Design review of the part built by this model. Coordinates are the model's own, in mm. A direction names the side the tool comes from. Give positions to 0.01 mm unless a question says otherwise; leave off trailing zeros. Write each loop counter-clockwise with the first axis right and the second up, starting at its lowest first coordinate (ties: lowest second). Pieces come first, ordered by that corner, then holes. Notation, with made-up numbers: M 26,16 L 48,16 A9 cw 48,21 Z; hole C 76,74.25 d10. An arc over 180 degrees is marked long. Answer in a Markdown table with one row per item.
```python
from build123d import *

# Parameters (mm, degrees)
BOSS_EXTRUDE4_DEPTH  = 1.5
SKETCH5_W            = 205
SKETCH5_H            = 54
BOSS_EXTRUDE5_DEPTH  = 1.5
SKETCH8_W            = 1.5
SKETCH8_H            = 430
BOSS_EXTRUDE14_DEPTH = 4
SKETCH7_W            = 205
SKETCH7_H            = 54
BOSS_EXTRUDE18_DEPTH = 1.5
SKETCH9_W            = 433
SKETCH9_H            = 54
BOSS_EXTRUDE19_DEPTH = 1.5
SKETCH10_R           = 2.1
CUT_EXTRUDE1_DEPTH   = 10
CUT_EXTRUDE2_START   = -10
SKETCH17_R           = 2.1
CUT_EXTRUDE2_DEPTH   = 10
SKETCH16_R           = 2.1
CUT_EXTRUDE3_DEPTH   = 10
CUT_EXTRUDE4_START   = -10
SKETCH11_R           = 2.1
CUT_EXTRUDE4_DEPTH   = 10
SKETCH12_R           = 2.1
CUT_EXTRUDE5_DEPTH   = 10
SKETCH13_R           = 2.1
CUT_EXTRUDE6_DEPTH   = 10
CUT_EXTRUDE7_START   = -10
SKETCH14_R           = 2.1
CUT_EXTRUDE7_DEPTH   = 10
CUT_EXTRUDE8_START   = -10
SKETCH15_R           = 2.1
CUT_EXTRUDE8_DEPTH   = 10
SKETCH18_W           = 41
SKETCH18_H           = 21.003646253
CUT_EXTRUDE9_DEPTH   = 10
SKETCH21_W           = 53
SKETCH21_H           = 58
CUT_EXTRUDE12_DEPTH  = 10
SKETCH23_W           = 7
SKETCH23_H           = 18
CUT_EXTRUDE14_DEPTH  = 31
SKETCH24_W           = 7
SKETCH24_H           = 18
CUT_EXTRUDE15_DEPTH  = 31


with BuildPart() as part:
    # Sketch4 → Boss-Extrude4 (new body)
    with BuildSketch(Plane(origin=(0, 0, 0), x_dir=(1, 0, 0), z_dir=(0, 1, 0))):
        Polygon((124.01347733, 430), (329.01347733, 430), (329.01347733, 0), (124.01347733, 0), (124.01347733, 200), (124.01347733, 365), align=None)
    extrude(amount=BOSS_EXTRUDE4_DEPTH)

    # Sketch5 → Boss-Extrude5 (add)
    with BuildSketch(Plane.XY):
        with Locations((226.51347733, -25.5)):
            Rectangle(SKETCH5_W, SKETCH5_H)
    extrude(amount=BOSS_EXTRUDE5_DEPTH)

    # Sketch8 → Boss-Extrude14 (add)
    with BuildSketch(Plane(origin=(0, 1.5, 0), x_dir=(1, 0, 0), z_dir=(0, 1, 0))):
        with Locations((328.26347733, 215)):
            Rectangle(SKETCH8_W, SKETCH8_H)
    extrude(amount=BOSS_EXTRUDE14_DEPTH)

    # Sketch7 → Boss-Extrude18 (add)
    with BuildSketch(Plane(origin=(0, 0, -430), x_dir=(-1, 0, 0), z_dir=(0, 0, -1))):
        with Locations((-226.51347733, -25.5)):
            Rectangle(SKETCH7_W, SKETCH7_H)
    extrude(amount=BOSS_EXTRUDE18_DEPTH)

    # Sketch9 → Boss-Extrude19 (add)
    with BuildSketch(Plane.ZY.offset(-124.01347733)):
        with Locations((-215, -25.5)):
            Rectangle(SKETCH9_W, SKETCH9_H)
    extrude(amount=BOSS_EXTRUDE19_DEPTH)

    # Sketch10 → Cut-Extrude1 (cut)
    with BuildSketch(Plane(origin=(0, 0, -431.5), x_dir=(-1, 0, 0), z_dir=(0, 0, -1))):
        with Locations((-154.01347733, -42.5)):
            Circle(SKETCH10_R)
    extrude(amount=-CUT_EXTRUDE1_DEPTH, mode=Mode.SUBTRACT)

    # Sketch17 → Cut-Extrude2 (cut)
    with BuildSketch(Plane.XY.offset(1.5).offset(CUT_EXTRUDE2_START)):
        with Locations(Location((154.01347733, -42.5, 0), (0, 0, 180))):
            Circle(SKETCH17_R)
    extrude(amount=CUT_EXTRUDE2_DEPTH, mode=Mode.SUBTRACT)

    # Sketch16 → Cut-Extrude3 (cut)
    with BuildSketch(Plane.XY.offset(1.5)):
        with Locations((134.023652304, -42.521836229)):
            Circle(SKETCH16_R)
    extrude(amount=-CUT_EXTRUDE3_DEPTH, mode=Mode.SUBTRACT)

    # Sketch11 → Cut-Extrude4 (cut)
    with BuildSketch(Plane(origin=(0, 0, -431.5), x_dir=(-1, 0, 0), z_dir=(0, 0, -1)).offset(CUT_EXTRUDE4_START)):
        with Locations(Location((-134.023652304, -42.521836229, 0), (0, 0, 180))):
            Circle(SKETCH11_R)
    extrude(amount=CUT_EXTRUDE4_DEPTH, mode=Mode.SUBTRACT)

    # Sketch12 → Cut-Extrude5 (cut)
    with BuildSketch(Plane(origin=(0, 0, -431.5), x_dir=(-1, 0, 0), z_dir=(0, 0, -1))):
        with Locations((-134.017306734, -22.477341223)):
            Circle(SKETCH12_R)
    extrude(amount=-CUT_EXTRUDE5_DEPTH, mode=Mode.SUBTRACT)

    # Sketch13 → Cut-Extrude6 (cut)
    with BuildSketch(Plane(origin=(0, 0, -431.5), x_dir=(-1, 0, 0), z_dir=(0, 0, -1))):
        with Locations((-154.003183789, -22.514424589)):
            Circle(SKETCH13_R)
    extrude(amount=-CUT_EXTRUDE6_DEPTH, mode=Mode.SUBTRACT)

    # Sketch14 → Cut-Extrude7 (cut)
    with BuildSketch(Plane.XY.offset(1.5).offset(CUT_EXTRUDE7_START)):
        with Locations(Location((134.017306734, -22.477341223, 0), (0, 0, 180))):
            Circle(SKETCH14_R)
    extrude(amount=CUT_EXTRUDE7_DEPTH, mode=Mode.SUBTRACT)

    # Sketch15 → Cut-Extrude8 (cut)
    with BuildSketch(Plane.XY.offset(1.5).offset(CUT_EXTRUDE8_START)):
        with Locations(Location((154.003183789, -22.514424589, 0), (0, 0, 180))):
            Circle(SKETCH15_R)
    extrude(amount=CUT_EXTRUDE8_DEPTH, mode=Mode.SUBTRACT)

    # Sketch18 → Cut-Extrude9 (cut)
    with BuildSketch(Plane(origin=(0, 1.5, 0), x_dir=(1, 0, 0), z_dir=(0, 1, 0))):
        with Locations((144.235269619, 254.779446877)):
            Rectangle(SKETCH18_W, SKETCH18_H)
    extrude(amount=-CUT_EXTRUDE9_DEPTH, mode=Mode.SUBTRACT)

    # Sketch21 → Cut-Extrude12 (cut)
    with BuildSketch(Plane(origin=(0, 1.5, 0), x_dir=(1, 0, 0), z_dir=(0, 1, 0))):
        with Locations((190.51347733, 360.765424222)):
            Rectangle(SKETCH21_W, SKETCH21_H)
    extrude(amount=-CUT_EXTRUDE12_DEPTH, mode=Mode.SUBTRACT)

    # Sketch23 → Cut-Extrude14 (cut)
    with BuildSketch(Plane.XY.offset(1.5)):
        with Locations((325.51347733, -3.5)):
            Rectangle(SKETCH23_W, SKETCH23_H)
    extrude(amount=-CUT_EXTRUDE14_DEPTH, mode=Mode.SUBTRACT)

    # Sketch24 → Cut-Extrude15 (cut)
    with BuildSketch(Plane(origin=(0, 0, -431.5), x_dir=(-1, 0, 0), z_dir=(0, 0, -1))):
        with Locations((-325.51347733, -3.5)):
            Rectangle(SKETCH24_W, SKETCH24_H)
    extrude(amount=-CUT_EXTRUDE15_DEPTH, mode=Mode.SUBTRACT)


solid = part.part
```
1) Insertion check: P1, Ø5, axis at y = -3, z = -56.5, coming from the +X side; P2, Ø15.5, axis at y = -7, z = -422.5, coming from the +X side; P3, Ø5, axis at x = 241.5, z = -65, coming from the +Y side. Each pin has a flat end and moves straight along its axis. Give the tip position at first contact, or say it passes through.
Geometry says:
| item | result |
|---|---|
| P1 | x = 124.01 |
| P2 | x = 322.01 |
| P3 | y = 1.5 |
2) The part is to be moulded in two halves that separate along Z. For faces 6 (the face through (227, -26, 1.5)), 7 (the face through (124.013, -26, -218)), 8 (the face through (226, 1.5, -218)), say which applies: released by +Z, released by -Z, zero draft, split by the parting line, or undercut.
Geometry says:
| item | result |
|---|---|
| face 6 | released by +Z |
| face 7 | undercut |
| face 8 | zero draft |
3) Add section D-D (y = -4.5). Write out the cut boundary in (x, z), and give its area (3 significant figures).
Geometry says:
| item | result |
|---|---|
| outline | M 122.51,-431.5 L 322.01,-431.5 L 322.01,-430 L 124.01,-430 L 124.01,-265.28 L 123.74,-265.28 L 123.74,-244.28 L 124.01,-244.28 L 124.01,0 L 322.01,0 L 322.01,1.5 L 122.51,1.5 Z |
| area | 1,240 mm^2 |
4) Add section A-A (x = 199). Write out the cut boundary in (y, z).
Geometry says:
| item | result |
|---|---|
| outline | M -52.5,-431.5 L 1.5,-431.5 L 1.5,-389.77 L 0,-389.77 L 0,-430 L -52.5,-430 Z; M -52.5,0 L 0,0 L 0,-331.77 L 1.5,-331.77 L 1.5,1.5 L -52.5,1.5 Z |
5) Add section B-B (x = 230). Write out the cut boundary in (y, z), and give its area (3 significant figures).
Geometry says:
| item | result |
|---|---|
| outline | M -52.5,-431.5 L 1.5,-431.5 L 1.5,1.5 L -52.5,1.5 L -52.5,0 L 0,0 L 0,-430 L -52.5,-430 Z |
| area | 807 mm^2 |
6) Add section C-C (z = -217). Write out the cut boundary in (x, y), and give its area (4 significant figures).
Geometry says:
| item | result |
|---|---|
| outline | M 122.51,-52.5 L 124.01,-52.5 L 124.01,0 L 329.01,0 L 329.01,5.5 L 327.51,5.5 L 327.51,1.5 L 122.51,1.5 Z |
| area | 394.5 mm^2 |
7) To check wall thickness, follow probe 1 along Z at (x, y) = (208.5, -5); probe 2 along X at (y, z) = (0.5, -373.5); probe 3 along Y at (x, z) = (134.5, -210.5). State the ranges of each line that lie inside material, in increasing order. Write a range as [from, to].
Geometry says:
| item | result |
|---|---|
| probe 1 | [-431.5, -430], [0, 1.5] |
| probe 2 | [122.51, 164.01], [217.01, 329.01] |
| probe 3 | [0, 1.5] |
8) For faces 1 (the face through (122.513, -25, -218)), 2 (the face through (228, 0, -218)), 3 (the face through (322.013, 0.2, -10.5)), 4 (the face through (322.013, 0.2, -419.5)), 5 (the face through (227, -26, -431.5)), list the 3-axis set-ups (+Z, -Z, +X, -X, +Y, -Y) from which the entire face can be reached by the end or side of a thin tool; tool diameter is ignored.
Geometry says:
| item | result |
|---|---|
| face 1 | +Z, -Z, -X, +Y, -Y |
| face 2 | +X, -Y |
| face 3 | +Z, +X, +Y |
| face 4 | -Z, +X, +Y |
| face 5 | -Z, +X, -X, +Y, -Y |
